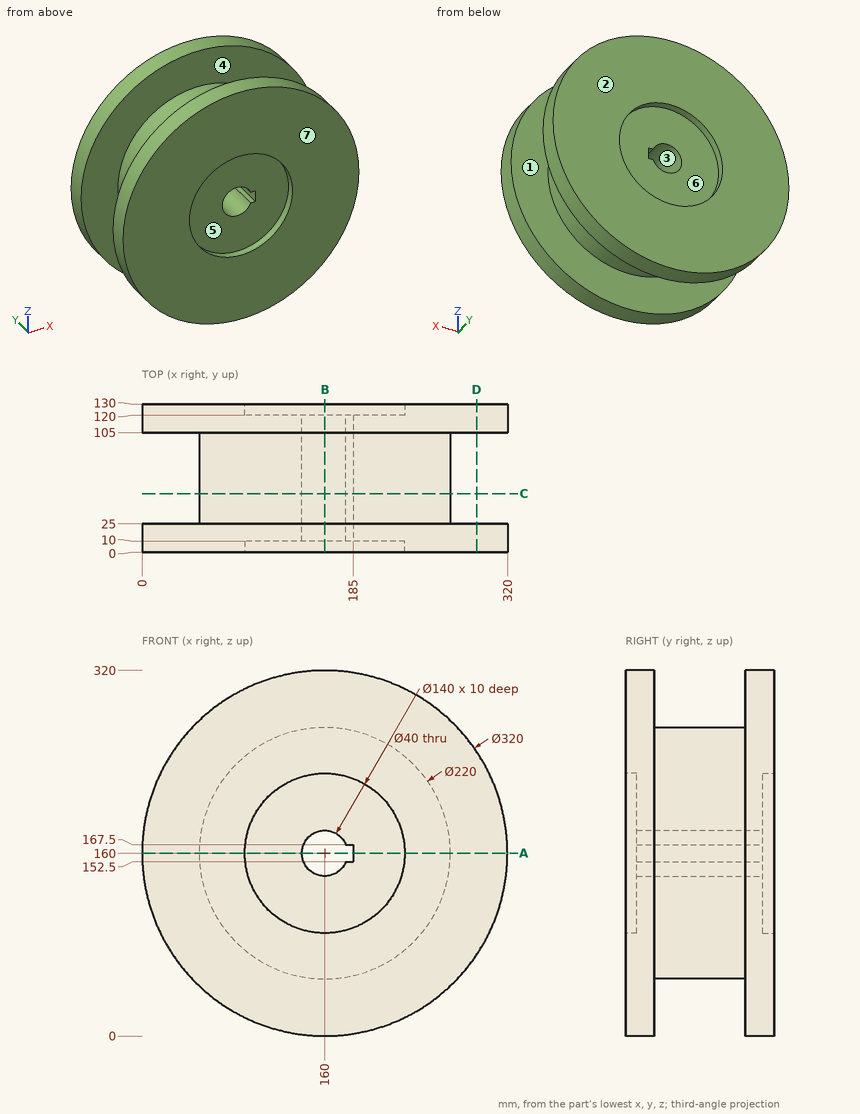
Verification items for this drawing (mm, ordinates from the low corner). A direction names the side the tool comes from. Give positions to 0.01 mm unless a question says otherwise; leave off trailing zeros. Loops run counter-clockwise (first coordinate to the right, second up) from the corner with the lowest first, then second, coordinate; pieces in that order, holes last.
(1) Section check A-A on z = 160. Record the cut outline in (x, y).
From the geometry:
outline: (0, 0) - (90, 0) - (90, 10) - (140, 10) - (140, 120) - (90, 120) - (90, 130) - (0, 130) - (0, 105) - (50, 105) - (50, 25) - (0, 25) - close; (185, 10) - (230, 10) - (230, 0) - (320, 0) - (320, 25) - (270, 25) - (270, 105) - (320, 105) - (320, 130) - (230, 130) - (230, 120) - (185, 120) - close
(2) Thickness scan on L1, parallel to Y at x = 256.5, z = 41; L2, parallel to Z at x = 160, y = 70; L3, parallel to Y at x = 193, z = 173.5. Record the ranges inside material, lowest first.
From the geometry:
L1: y = 0 to 25, 105 to 130
L2: z = 50 to 140, 180 to 270
L3: y = 10 to 120
(3) Section check C-C on y = 51.5. Record the cut outline in (x, z).
From the geometry:
outline: circle Ø220 at (160, 160); hole (178.54, 152.5) - (185, 152.5) - (185, 167.5) - (178.54, 167.5) arc R20 ccw (long way) to start
(4) Release check for a two-part mould opening along Y. For the marked faces 1, 2, 3 and 4 record: released by +Y, released by -Y, zero draft, split by the parting line, or undercut.
From the geometry:
face 1: undercut
face 2: released by +Y
face 3: zero draft
face 4: undercut
(5) Set-up check for the marked faces 5, 6 and 7: record each of +Z, -Z, +X, -X, +Y, -Y from which the full face is reachable in a straight line by a thin tool's end or side.
From the geometry:
face 5: -Y
face 6: +Y
face 7: +Z, -Z, +X, -X, -Y
(6) Section check D-D on x = 293. Record the cut outline in (y, z), then the cut area to 3 significant figures.
From the geometry:
outline: (0, 71.06) - (25, 71.06) - (25, 248.94) - (0, 248.94) - close; (105, 71.06) - (130, 71.06) - (130, 248.94) - (105, 248.94) - close
area: 8,890 mm2
(7) Section check B-B on x = 160. Record the cut outline in (y, z).
From the geometry:
outline: (0, 0) - (25, 0) - (25, 50) - (105, 50) - (105, 0) - (130, 0) - (130, 90) - (120, 90) - (120, 140) - (10, 140) - (10, 90) - (0, 90) - close; (0, 230) - (10, 230) - (10, 180) - (120, 180) - (120, 230) - (130, 230) - (130, 320) - (105, 320) - (105, 270) - (25, 270) - (25, 320) - (0, 320) - close
(8) Depth check by flat-ended pin: pin 1 Ø2 at (x, y) = (100.5, 59) entering from -Z; pin 2 Ø12 at (y, z) = (63, 156.5) entering from -X; pin 3 Ø10 at (x, y) = (45, 27) entering from -Z. Enter the tip coordinate at first touch or a pass-through.
From the geometry:
pin 1: stops at z = 66.85
pin 2: stops at x = 50
pin 3: stops at z = 44.21
